```python
from build123d import *

# Parameters (mm, degrees)
EXTRUDE_1_DEPTH          = 4.4
CUT_EXTRUDE_1_DEPTH      = 0.6
FILLET_1_R               = 1.5
CUT_EXTRUDE_2_DEPTH      = 53.909660275
CUT_EXTRUDE_2_DEPTH_BACK = 53.909660275


with BuildPart() as part:
    # 스케치1 → 보스-돌출1 (new body)
    with BuildSketch(Plane(origin=(0, 0, 0), x_dir=(1, 0, 0), z_dir=(0, 1, 0))):
        Polygon((27.293187568, -27.293187568), (37.283187568, -9.99), (37.283187568, 9.99), (27.293187568, 27.293187568), (9.99, 37.283187568), (-9.99, 37.283187568), (-27.293187568, 27.293187568), (-37.283187568, 9.99), (-37.283187568, -9.99), (-27.293187568, -27.293187568), (-9.99, -37.283187568), (9.99, -37.283187568), align=None)
    extrude(amount=EXTRUDE_1_DEPTH)

    # 스케치2 → 컷-돌출1 (cut)
    with BuildSketch(Plane(origin=(0, 4.4, 0), x_dir=(1, 0, 0), z_dir=(0, 1, 0))):
        Polygon((-26.120860153, 26.120860153), (-35.681758538, 9.560898385), (-35.681758538, -9.560898385), (-26.120860153, -26.120860153), (-9.560898385, -35.681758538), (9.560898385, -35.681758538), (26.120860153, -26.120860153), (35.681758538, -9.560898385), (35.681758538, 9.560898385), (26.120860153, 26.120860153), (9.560898385, 35.681758538), (-9.560898385, 35.681758538), align=None)
        Polygon((24.656758538, -24.656758538), (33.681758538, -9.025), (33.681758538, 9.025), (24.656758538, 24.656758538), (9.025, 33.681758538), (-9.025, 33.681758538), (-24.656758538, 24.656758538), (-33.681758538, 9.025), (-33.681758538, -9.025), (-24.656758538, -24.656758538), (-9.025, -33.681758538), (9.025, -33.681758538), align=None, mode=Mode.SUBTRACT)
    cut_extrude_1 = extrude(amount=-CUT_EXTRUDE_1_DEPTH, mode=Mode.SUBTRACT)

    # 필렛1
    fillet_1_edges = [part.edges().sort_by_distance(p)[0] for p in [
        (0, 0, 37.283187568),
        (-18.641593784, 0, 32.288187568),
        (37.283187568, 4.4, 0),
        (-32.288187568, 0, 18.641593784),
        (-37.283187568, 0, 0),
        (-32.288187568, 0, -18.641593784),
        (-18.641593784, 0, -32.288187568),
        (0, 0, -37.283187568),
        (18.641593784, 0, -32.288187568),
        (32.288187568, 0, -18.641593784),
        (37.283187568, 0, 0),
        (32.288187568, 0, 18.641593784),
        (18.641593784, 0, 32.288187568),
        (32.288187568, 4.4, -18.641593784),
        (18.641593784, 4.4, -32.288187568),
        (0, 4.4, -37.283187568),
        (-18.641593784, 4.4, -32.288187568),
        (-32.288187568, 4.4, -18.641593784),
        (-37.283187568, 4.4, 0),
        (-32.288187568, 4.4, 18.641593784),
        (-18.641593784, 4.4, 32.288187568),
        (0, 4.4, 37.283187568),
        (18.641593784, 4.4, 32.288187568),
        (32.288187568, 4.4, 18.641593784),
    ]]
    fillet(fillet_1_edges, radius=FILLET_1_R)

    # 스케치3 → 컷-돌출2 (cut, two sides: drawn at the far end of the back side and taken through both)
    with BuildSketch(Plane(origin=(0, 4.4, 0), x_dir=(1, 0, 0), z_dir=(0, 1, 0)).offset(-CUT_EXTRUDE_2_DEPTH_BACK)):
        Polygon((23.778297569, 23.778297569), (8.703460969, 32.481758538), (-8.703460969, 32.481758538), (-23.778297569, 23.778297569), (-32.481758538, 8.703460969), (-32.481758538, -8.703460969), (-23.778297569, -23.778297569), (-8.703460969, -32.481758538), (8.703460969, -32.481758538), (23.778297569, -23.778297569), (32.481758538, -8.703460969), (32.481758538, 8.703460969), align=None)
    extrude(amount=CUT_EXTRUDE_2_DEPTH + CUT_EXTRUDE_2_DEPTH_BACK, mode=Mode.SUBTRACT)

    # 대칭 복사1: 컷-돌출1 across plane
    add(cut_extrude_1.mirror(Plane.ZX.offset(2.2)), mode=Mode.SUBTRACT)


solid = part.part
```
The listing builds one solid part. Answer for the finished solid, in the listing's coordinates (mm). A direction names the side the tool comes from. Coordinates: 2 decimals unless noted, no trailing zeros. Write each loop counter-clockwise with the first axis right and the second up, starting at its lowest first coordinate (ties: lowest second). Pieces come first, ordered by that corner, then holes. Notation, with made-up numbers: (-14.5, 32.5) - (3.5, 32.5) arc R17 cw to (3.5, 45.5) - close; hole circle Ø10 at (85.25, 3). An arc over 180 degrees is marked (long way). Return JSON: item names as keys, results as strings. Group by question number.
1. Straight lines are drawn through the part: L1, parallel to X at y = 2.05, z = 1.5; L2, parallel to Z at x = -12.5, y = 0.5; L3, parallel to Z at x = 16.5, y = 2.8. For each, find the intervals that lie inside material, in ascending order.
2. A cutting plane is placed at B-B, the plane x = -3. Determine the outline of the cut face in (y, z), plus the area to 3 significant figures.
3. A cutting plane is placed at A-A, the plane z = 4.5. Determine the outline of the cut face in (x, y), plus the area to 3 significant figures.
4. Which of the six approach directions +Z, -Z, +X, -X, +Y, -Y give full straight-line access (tool end or side, diameter ignored) to faces 5 (the flat face through (29.232, 4.104, -16.731)), 6 (the flat face through (-32.482, 2, 0)), 7 (the flat face through (16.731, 0.296, 29.232)), 8 (the flat face through (32.22, 2.19, 18.76))?
5. Given pin 1 (1.5 mm diameter, centred on y = 3.5, z = 16.5, fed in from +X); pin 2 (0.7 mm diameter, centred on y = 0.5, z = -3.5, fed in from +X); pin 3 (0.7 mm diameter, centred on y = 4, z = 2.5, fed in from -X), each flat-ended and moving along its own axis, determine where each tip first touches the part or whether it passes through.
6. Determine the mould class of faces 1 (the flat face through (17.957, 4.104, -30.834)), 2 (the flat face through (28.19, 2.17, -16.14)), 3 (the cylindrical face through (-31.97, 0.43, -18.29)), 4 (the flat face through (18.76, 2.19, -32.22)) for opening direction X: released by +X, released by -X, zero draft, split by the parting line, or undercut.
Ans:
{
 "1": {"L1": "-37.28 to -32.48, 32.48 to 37.28", "L2": "-35.39 to -33.98, -31.68 to -30.29, 30.29 to 31.68, 33.98 to 35.39", "L3": "-33.52 to -27.98, 27.98 to 33.52"},
 "2": {"outline": "(0, -35.78) arc R1.5 ccw to (1.5, -37.28) - (2.9, -37.28) arc R1.5 ccw to (4.4, -35.78) - (4.4, -35.68) - (3.8, -35.68) - (3.8, -33.68) - (4.4, -33.68) - (4.4, -32.48) - (0, -32.48) - (0, -33.68) - (0.6, -33.68) - (0.6, -35.68) - (0, -35.68) - close; (0, 32.48) - (4.4, 32.48) - (4.4, 33.68) - (3.8, 33.68) - (3.8, 35.68) - (4.4, 35.68) - (4.4, 35.78) arc R1.5 ccw to (2.9, 37.28) - (1.5, 37.28) arc R1.5 ccw to (0, 35.78) - (0, 35.68) - (0.6, 35.68) - (0.6, 33.68) - (0, 33.68) - close", "area": "35.5 mm²"},
 "3": {"outline": "(-37.28, 1.5) arc R1.5 ccw to (-35.78, 0) - (-35.68, 0) - (-35.68, 0.6) - (-33.68, 0.6) - (-33.68, 0) - (-32.48, 0) - (-32.48, 4.4) - (-33.68, 4.4) - (-33.68, 3.8) - (-35.68, 3.8) - (-35.68, 4.4) - (-35.78, 4.4) arc R1.5 ccw to (-37.28, 2.9) - close; (32.48, 0) - (33.68, 0) - (33.68, 0.6) - (35.68, 0.6) - (35.68, 0) - (35.78, 0) arc R1.5 ccw to (37.28, 1.5) - (37.28, 2.9) arc R1.5 ccw to (35.78, 4.4) - (35.68, 4.4) - (35.68, 3.8) - (33.68, 3.8) - (33.68, 4.4) - (32.48, 4.4) - close", "area": "35.5 mm²"},
 "4": {"face 5": "+Y", "face 6": "+Y, -Y", "face 7": "-Y", "face 8": "+Z, +X, +Y, -Y"},
 "5": {"pin 1": "x = 33.89", "pin 2": "x = 37.14", "pin 3": "x = -37.08"},
 "6": {"face 1": "undercut", "face 2": "undercut", "face 3": "released by -X", "face 4": "released by +X"}
}
